```python
from build123d import *

# Parameters (mm, degrees)
F0_W     = 380
F0_H     = 380
F1_DEPTH = 350
F2_W     = 342
F2_H     = 312
F3_DEPTH = 361
F4_W     = 40
F4_H     = 40
F5_DEPTH = 150


with BuildPart() as f1:
    # F0 (on Top) → F1 (new body)
    with BuildSketch(Plane.XY):
        Rectangle(F0_W, F0_H)
    extrude(amount=F1_DEPTH)

    # F2 (on face) → F3 (cut)
    with BuildSketch(Plane.XZ.offset(190)):
        with Locations((0, 175)):
            Rectangle(F2_W, F2_H)
    extrude(amount=-F3_DEPTH, mode=Mode.SUBTRACT)

    # F4 (on face) → F5 (join)
    with BuildSketch(Plane(origin=(0, 0, 0), x_dir=(1, 0, 0), z_dir=(0, 0, -1))):
        with Locations((170, 170)):
            Rectangle(F4_W, F4_H)
        with Locations((-170, 170)):
            Rectangle(F4_W, F4_H)
        with Locations((-170, -170)):
            Rectangle(F4_W, F4_H)
        with Locations((170, -170)):
            Rectangle(F4_W, F4_H)
    extrude(amount=F5_DEPTH)


solid = f1.part
```
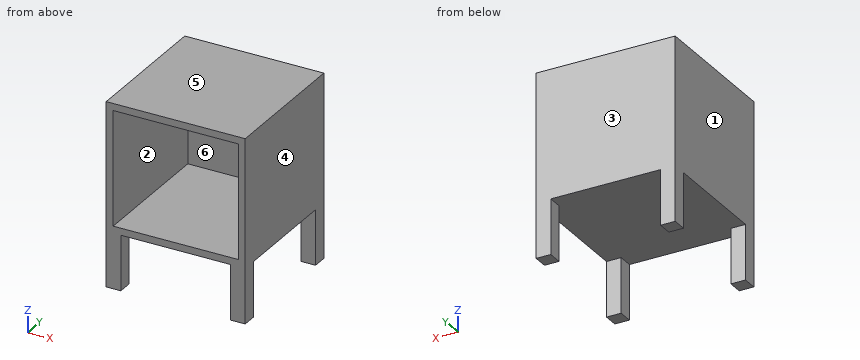
Can you work these out from the model? Positions are in its coordinate system, mm. Face numbers are marked on the shaded views. A direction names the side the tool comes from. Round coordinates to 2 decimals unless told otherwise and drop trailing zeros. Loops run counter-clockwise (first coordinate to the right, second up) from the corner with the lowest first, then second, coordinate; pieces in that order, holes last.
Item 1: Will these pins go through, and if not, where does the flat tip stop? pin 1 Ø8 at (x, y) = (-112.5, -119) entering from -Z; pin 2 Ø1 at (x, z) = (-146.5, 189.5) entering from -Y.
Item 2: Suppose I cut it at C-C, the plane x = 14. Write out the boundary of the cut face in (y, z).
Item 3: Which directions (+Z, -Z, +X, -X, +Y, -Y) give clear straight access to the entire face, cutting with the end or side of a thin tool? Please do the marked faces 5 and 6.
Item 4: Suppose I cut it at A-A, the plane z = -85. Write out the boundary of the cut face in (x, y), then the cut area to 3 significant figures.
Item 5: If we mould it in two halves opening along X, with no side actions, what happens to the marked faces 1, 2, 3 and 4? For each: +X half, -X half, draft (parallel to the pull), parting line (faces both ways), or undercut.
Item 6: Suppose I cut it at B-B, the plane y = 157.5. Write out the boundary of the cut face in (x, z), then the cut area to 3 significant figures.
Item 7: Please list where these lines run through material, in increasing order: L1, parallel to X at y = 69.5, z = 145; L2, parallel to X at y = -151, z = -63.5; L3, parallel to Z at x = 31, y = 112.5.
Item 8: Suppose I cut it at D-D, the plane z = 97. Write out the boundary of the cut face in (x, y).
Reported:
1. pin 1: stops at z = 0
1. pin 2: stops at y = 171
2. outline: (-190, 0) - (190, 0) - (190, 350) - (-190, 350) - (-190, 331) - (171, 331) - (171, 19) - (-190, 19) - close
3. face 5: +Z, +X, -X, +Y, -Y
3. face 6: -Y
4. outline: (-190, -190) - (-150, -190) - (-150, -150) - (-190, -150) - close; (-190, 150) - (-150, 150) - (-150, 190) - (-190, 190) - close; (150, -190) - (190, -190) - (190, -150) - (150, -150) - close; (150, 150) - (190, 150) - (190, 190) - (150, 190) - close
4. area: 6,400 mm2
5. face 1: -X half
5. face 2: undercut
5. face 3: draft
5. face 4: +X half
6. outline: (-190, -150) - (-150, -150) - (-150, 0) - (150, 0) - (150, -150) - (190, -150) - (190, 350) - (-190, 350) - close; hole (-171, 19) - (171, 19) - (171, 331) - (-171, 331) - close
6. area: 38,300 mm2
7. L1: x = -190 to -171, 171 to 190
7. L2: x = -190 to -150, 150 to 190
7. L3: z = 0 to 19, 331 to 350
8. outline: (-190, -190) - (-171, -190) - (-171, 171) - (171, 171) - (171, -190) - (190, -190) - (190, 190) - (-190, 190) - close
